Could you check a few things on this model? Use its own coordinates, in mm. Round coordinates to 2 decimals unless told otherwise and drop trailing zeros. Loops run counter-clockwise (first coordinate to the right, second up) from the corner with the lowest first, then second, coordinate; pieces in that order, holes last. Notation, with made-up numbers: (64.5, 81.25) -> (85.5, 81.25) arc R12 ccw to (85.5, 102.25) -> close; hole circle Ø3 at (-35.5, -4.5). An arc over 180 degrees is marked (long way). Put each result on its own line as item: value. Start each with the question number.
1. I need wall thicknesses on line 1 (Y direction, x = -1, z = 275); line 2 (Y direction, x = 6.25, z = 227); line 3 (Z direction, x = -1.25, y = 9). Which ranges of each line are inside material? Lowest first, please. Write a range as [from, to].
2. Imagine slicing it at B-B, the plane y = 28.5. Please give me the cut outline in (x, z).
3. I'm going to push flat-ended pins straight in: P1, Ø3, axis at x = 2, z = 264, coming from the -Y side; P2, Ø1, axis at x = -6.5, y = 107, coming from the -Z side; P3, Ø2, axis at x = 4, z = 117.5, coming from the -Y side. Where does each tip first touch, or does it pass through?
4. Imagine slicing it at A-A, the plane z = 21. Please give me the cut outline in (x, y), and give its area (3 significant figures).
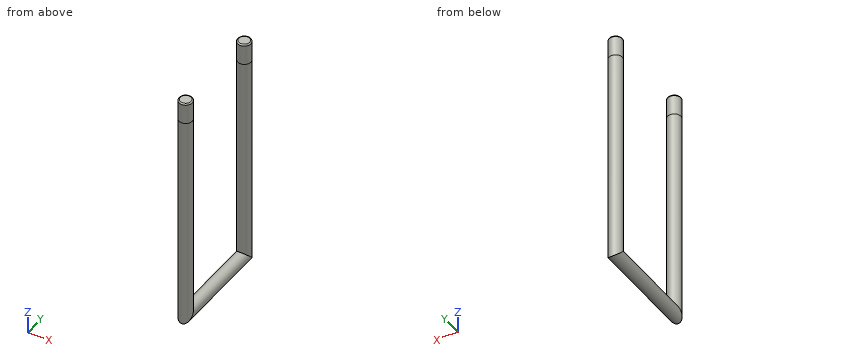
```python
from build123d import *

# Parameters (mm, degrees)
SKETCH_1_R                 = 11
EXTRUDE_1_DEPTH            = 352
SKETCH_2_R                 = 11
EXTRUDE_2_DEPTH            = 158
PATTERN_LINEAR_1_OUTLINE_R = 11
PATTERN_LINEAR_1_DEPTH     = 352
SKETCH_3_R                 = 10.9995
EXTRUDE_3_DEPTH            = 35
CHAMFER_1_SIZE             = 21.999
FILLET_1_R                 = 2


with BuildPart() as part:
    # 草图1 → 拉伸1 (new body)
    with BuildSketch(Plane.XY):
        Circle(SKETCH_1_R)
    extrude(amount=EXTRUDE_1_DEPTH)

    # 草图2 → 拉伸2 (add)
    with BuildSketch(Plane(origin=(0, 0, 0), x_dir=(1, 0, 0), z_dir=(0, 1, 0))):
        with Locations(Location((0, 0, 0), (0, 0, 180))):
            Circle(SKETCH_2_R)
    extrude(amount=EXTRUDE_2_DEPTH)


with BuildPart() as pattern_linear_1_tool:
    # 阵列(线性)1: read off the stored shape, not the designer's step
    # 阵列(线性)1 outline → 阵列(线性)1 (new body)
    with BuildSketch(Plane.XY):
        with Locations((0, 158)):
            Circle(PATTERN_LINEAR_1_OUTLINE_R)
    extrude(amount=PATTERN_LINEAR_1_DEPTH)


with BuildPart() as part_1:
    add(part.part)


with BuildPart() as part_2:
    # 阵列(线性)1: joined with pattern_linear_1_tool
    add(part_1.part.fuse(pattern_linear_1_tool.part, tol=0.00001))

    # 草图3 → 拉伸3 (add)
    with BuildSketch(Plane.XY.offset(352)):
        with Locations((0, 158)):
            Circle(SKETCH_3_R)
        Circle(SKETCH_3_R)
    extrude(amount=EXTRUDE_3_DEPTH)

    # 倒角1
    # the kernel refuses this chamfer: 21.999 mm, written as the material it adds along each edge
    with BuildSketch(Plane(origin=(67.574454052, 0, 0), x_dir=(0, -1, 0), z_dir=(-1, 0, 0))) as chamfer_1_piece_1_section:
        Polygon((CHAMFER_1_SIZE, 0), (0, -CHAMFER_1_SIZE), (0, 0), align=None)
    chamfer_1_piece_1 = extrude(amount=135.148908105, mode=Mode.PRIVATE)
    chamfer_1_piece_1 = chamfer_1_piece_1 & Plane(origin=(0, 0, 0), x_dir=(1, 0, 0), z_dir=(0, 0, -1)) * Cylinder(11, 359, mode=Mode.PRIVATE)
    chamfer_1_piece_1 = chamfer_1_piece_1 & Plane(origin=(0, 0, 0), x_dir=(-1, 0, 0), z_dir=(0, -1, 0)) * Cylinder(11, 359, mode=Mode.PRIVATE)
    add(chamfer_1_piece_1)
    with BuildSketch(Plane(origin=(-67.574454052, 158, 0), x_dir=(0, 0, -1), z_dir=(1, 0, 0))) as chamfer_1_piece_2_section:
        Polygon((CHAMFER_1_SIZE, 0), (0, CHAMFER_1_SIZE), (0, 0), align=None)
    chamfer_1_piece_2 = extrude(amount=135.148908105, mode=Mode.PRIVATE)
    chamfer_1_piece_2 = chamfer_1_piece_2 & Plane(origin=(0, 158, 0), x_dir=(-1, 0, 0), z_dir=(0, -1, 0)) * Cylinder(11, 359, mode=Mode.PRIVATE)
    chamfer_1_piece_2 = chamfer_1_piece_2 & Plane(origin=(0, 158, 0), x_dir=(1, 0, 0), z_dir=(0, 0, -1)) * Cylinder(11, 359, mode=Mode.PRIVATE)
    add(chamfer_1_piece_2)

    # 圆角1
    fillet_1_edges = [part_2.edges().sort_by_distance(p)[0] for p in [
        (-10.9995, 158, 387),
        (-10.9995, 0, 387),
    ]]
    fillet(fillet_1_edges, radius=FILLET_1_R)


solid = part_2.part
```
Entries:
1. line 1: [-10.95, 10.95], [147.05, 168.95]
1. line 2: [-9.05, 9.05], [148.95, 167.05]
1. line 3: [-10.93, 387]
2. outline: circle Ø22 at (0, 0)
3. P1: y = -10.99
3. P2: z = -9.22
3. P3: y = -10.58
4. outline: circle Ø22 at (0, 0); circle Ø22 at (0, 158)
4. area: 760 mm^2
